Work out the finished part from the listing and answer in its coordinate system (mm). A direction names the side the tool comes from. Coordinates: 2 decimals unless noted, no trailing zeros. Order: outer loops, then holes, each group sorted by start corner. A loop starts at its lowest first (then second) coordinate and runs counter-clockwise, first axis right, second up. Notation, with made-up numbers: (13, 54.5) -> (42, 54.5) arc R29 cw to (42, 89.5) -> close; hole circle Ø3 at (29.25, -12). An arc over 180 degrees is marked (long way). Write item = value, one per line. Start each with the question number.
Q1. For a pull along X with two mould halves and no side action, classify faces 3 (the flat face through (11.8, 103.18, 2.46)), 4 (the flat face through (-1, 96, 5)), 5 (the cylindrical face through (103.103, 210.698, 2.535)) as +X half, -X half, draft (parallel to the pull), parting line (faces both ways), or undercut.
Q2. The part is cut by section B-B, the plane y = -18. Determine the outline of the cut face in (x, z).
Q3. Flat-ended cylindrical pins translate along their axes: pin 1 (1 mm diameter, centred on y = 176.5, z = 1.5, fed in from -X); pin 2 (3 mm diameter, centred on y = 60.5, z = 1, fed in from +X). Find the tip coordinate at first contact, or state that the pin passes through.
Q4. Straight lines are drawn through the part: L1, parallel to X at y = -7.5, z = 3.55; L2, parallel to Y at x = 85, z = 4.75; L3, parallel to Y at x = 2, z = 1.55. For each, find the intervals that lie inside material, in ascending order. Write a range as from..to.
Q5. Which of the six approach directions +Z, -Z, +X, -X, +Y, -Y give full straight-line access (tool end or side, diameter ignored) to faces 1 (the cylindrical face through (-95.266, 11.935, 2.535)), 2 (the flat face through (-82.771, -13, 2))?
Q6. The part is cut by section C-C, the plane x = -80. Determine the outline of the cut face in (y, z).
Q7. The part is cut by section A-A, the plane z = 2.15. Determine the outline of the cut face in (x, y), plus the area to 3 significant figures.
```python
from build123d import *

# Parameters (mm, degrees)
BOSS_EXTRUDE1_DEPTH = 5
SKETCH2_R           = 5
CUT_EXTRUDE1_DEPTH  = 5
SKETCH3_R           = 5
CUT_EXTRUDE2_DEPTH  = 6


with BuildPart() as part:
    # Sketch1 → Boss-Extrude1 (new body)
    with BuildSketch(Plane.XY):
        Polygon((-97.771110706, 14.82204599), (-97.771110706, -41.391157445), (-82.771110706, -41.391157445), (-82.771110706, 8.608842555), (114.36092365, 205.740876911), (103.754321932, 216.347478628), align=None)
    extrude(amount=BOSS_EXTRUDE1_DEPTH)

    # Sketch2 → Cut-Extrude1 (cut)
    with BuildSketch(Plane.XY.offset(5)):
        with Locations((-90.271110706, -33.891157445)):
            Circle(SKETCH2_R)
        with BuildLine():
            ThreePointArc((-90.271110669, -41.391157445), (-95.574411596, -39.194458273), (-97.771110706, -33.891157321))
            Line((-97.771110706, -33.891157321), (-97.771110706, -41.391157445))
            Line((-97.771110706, -41.391157445), (-90.271110669, -41.391157445))
        make_face()
        with BuildLine():
            Line((-82.771110706, -41.391157445), (-82.771110706, -33.891157445))
            ThreePointArc((-82.771110706, -33.891157445), (-84.967809834, -39.194458291), (-90.271110669, -41.391157445))
            Line((-90.271110669, -41.391157445), (-82.771110706, -41.391157445))
        make_face()
        with Locations((103.754321932, 205.740876911)):
            Circle(SKETCH2_R)
        with BuildLine():
            Line((109.057622903, 211.044177658), (103.754321932, 216.347478628))
            Line((103.754321932, 216.347478628), (98.451021073, 211.04417777))
            ThreePointArc((98.451021073, 211.04417777), (103.754322011, 213.240876911), (109.057622903, 211.044177658))
        make_face()
        with BuildLine():
            Line((114.36092365, 205.740876911), (109.057622903, 211.044177658))
            ThreePointArc((109.057622903, 211.044177658), (110.683418456, 208.61100258), (111.254321932, 205.740876911))
            ThreePointArc((111.254321932, 205.740876911), (110.683418433, 202.870751185), (109.057622817, 200.437576078))
            Line((109.057622817, 200.437576078), (114.36092365, 205.740876911))
        make_face()
    extrude(amount=-CUT_EXTRUDE1_DEPTH, mode=Mode.SUBTRACT)

    # Sketch3 → Cut-Extrude2 (cut, through all)
    with BuildSketch(Plane.XY.offset(5)):
        with Locations((-90.271110706, 11.715444272)):
            Circle(SKETCH3_R)
    extrude(amount=-CUT_EXTRUDE2_DEPTH, mode=Mode.SUBTRACT)


solid = part.part
```
Model answer:
q1.face_3 = +X half
q1.face_4 = draft
q1.face_5 = undercut
q2.outline = (-97.77, 0) -> (-82.77, 0) -> (-82.77, 5) -> (-97.77, 5) -> close
q3.pin_1 = 63.41
q3.pin_2 = -29.38
q4.L1 = -97.77..-82.77
q4.L2 = 176.38..197.59
q4.L3 = 93.38..114.59
q5.face_1 = +Z, -Z
q5.face_2 = +Z, -Z, +X, -Y
q6.outline = (11.38, 0) -> (32.59, 0) -> (32.59, 5) -> (11.38, 5) -> close
q7.outline = (-97.77, -33.89) arc R7.5 ccw to (-82.77, -33.89) -> (-82.77, 8.61) -> (109.06, 200.44) arc R7.5 ccw to (98.45, 211.04) -> (-97.77, 14.82) -> close; hole circle Ø10 at (-90.27, -33.89); hole circle Ø10 at (-90.27, 11.72); hole circle Ø10 at (103.75, 205.74)
q7.area = 4,740 mm2
